```python
from build123d import *
from OCP.BRepFilletAPI import BRepFilletAPI_MakeChamfer

# Parameters (mm, degrees)
SM_BASE_FLANGE_1_DEPTH = 60
CHAMFER_2_SIZE         = 35
CHAMFER_2_SIZE2        = 15
CHAMFER_3_SIZE         = 15
CHAMFER_3_SIZE2        = 35


# Sheet-metal steps are written as plain solids
with BuildPart() as part:
    # Sketch 1 → 基体-法兰1 (new body)
    with BuildSketch(Plane(origin=(0, 0, 0), x_dir=(0, 0, -1), z_dir=(1, 0, 0))):
        with BuildLine():
            Line((-50, -25), (-27.343145751, -2.343145751))
            ThreePointArc((-27.343145751, -2.343145751), (-24.74775896, -0.60896374), (-21.686291501, 0))
            Line((-21.686291501, 0), (21.686291501, 0))
            ThreePointArc((21.686291501, 0), (24.74775896, -0.60896374), (27.343145751, -2.343145751))
            Line((27.343145751, -2.343145751), (50, -25))
            Line((50, -25), (55.656854249, -19.343145751))
            Line((55.656854249, -19.343145751), (33, 3.313708499))
            ThreePointArc((33, 3.313708499), (27.809226419, 6.78207252), (21.686291501, 8))
            Line((21.686291501, 8), (-21.686291501, 8))
            ThreePointArc((-21.686291501, 8), (-27.809226419, 6.78207252), (-33, 3.313708499))
            Line((-33, 3.313708499), (-55.656854249, -19.343145751))
            Line((-55.656854249, -19.343145751), (-50, -25))
        make_face()
    extrude(amount=SM_BASE_FLANGE_1_DEPTH)

    # 倒角2
    chamfer_2_edges = [part.edges().sort_by_distance(p)[0] for p in [
        (60, -22.171572875, 52.828427125),
        (60, -22.171572875, -52.828427125),
    ]]
    chamfer_2_side = [part.faces().sort_by_distance(p)[0] for p in [
        (60, -8.83568579, 43.50745996),
    ]]
    chamfer(chamfer_2_edges, length=CHAMFER_2_SIZE, length2=CHAMFER_2_SIZE2, reference=chamfer_2_side[0])

    # 倒角3: one chamfer whose edges measure the first distance from different faces: ONE call of the kernel's chamfer builder (chamfer() names one face for all edges)
    chamfer_3_edges_1 = [part.edges().sort_by_distance(p)[0] for p in [
        (0, -22.171572875, 52.828427125),
    ]]
    chamfer_3_side_1 = [part.faces().sort_by_distance(p)[0] for p in [
        (22.5, -22.171572875, 52.828427125),
    ]]
    chamfer_3_edges_2 = [part.edges().sort_by_distance(p)[0] for p in [
        (0, -22.171572875, -52.828427125),
    ]]
    chamfer_3_side_2 = [part.faces().sort_by_distance(p)[0] for p in [
        (22.5, -22.171572875, -52.828427125),
    ]]
    chamfer_3 = BRepFilletAPI_MakeChamfer(part.part.solid().wrapped)
    for e in chamfer_3_edges_1:
        chamfer_3.Add(CHAMFER_3_SIZE, CHAMFER_3_SIZE2, e.wrapped, chamfer_3_side_1[0].wrapped)  # the first distance lies on this face
    for e in chamfer_3_edges_2:
        chamfer_3.Add(CHAMFER_3_SIZE, CHAMFER_3_SIZE2, e.wrapped, chamfer_3_side_2[0].wrapped)  # the first distance lies on this face
    add(Compound.cast(chamfer_3.Shape()), mode=Mode.REPLACE)


solid = part.part
```
The listing builds one solid part. Answer for the finished solid, in the listing's coordinates (mm). A direction names the side the tool comes from. Give positions to 0.01 mm unless a question says otherwise; leave off trailing zeros. Order: outer loops, then holes, each group sorted by start corner. A loop starts at its lowest first (then second) coordinate and runs counter-clockwise, first axis right, second up.
Item 1: Find the intervals of material crossed by probe 1 along Y at (x, z) = (5, -1.5); probe 2 along Z at (x, y) = (22.5, -12); probe 3 along Z at (x, y) = (24, -4.5), in increasing order.
From the geometry:
probe 1: y = 0 to 8
probe 2: z = -48.31 to -37, 37 to 48.31
probe 3: z = -40.81 to -29.5, 29.5 to 40.81
Item 2: The part is cut by section B-B, the plane y = -18. Give the vertices of the cut face in (x, z).
From the geometry:
outline: (10.76, -43) - (14.19, -54.31) - (45.81, -54.31) - (49.24, -43) - close; (10.76, 43) - (49.24, 43) - (45.81, 54.31) - (14.19, 54.31) - close
Item 3: For a pull along Z with two mould halves and no side action, classify faces 3 (the face through (60, 5, 0)), 4 (the face through (30, -22, 53)), 5 (the face through (30, -11, 36)) as pulls with the +Z half, pulls with the -Z half, needs draft (parallel to the pull), parting line crosses it, or undercut.
From the geometry:
face 3: needs draft
face 4: pulls with the +Z half
face 5: undercut
Item 4: Which of the six approach directions +Z, -Z, +X, -X, +Y, -Y give full straight-line access (tool end or side, diameter ignored) to faces 1 (the face through (30, 8, 0)), 2 (the face through (30, 0, 0))?
From the geometry:
face 1: +Z, -Z, +X, -X, +Y
face 2: +X, -X, -Y
Item 5: The part is cut by section A-A, the plane x = 22. Give the vertices of the cut face in (y, z), and give its area (3 significant figures).
From the geometry:
outline: (-25, -50) - (-19.34, -55.66) - (3.31, -33) arc R16 ccw to (8, -21.69) - (8, 21.69) arc R16 ccw to (3.31, 33) - (-19.34, 55.66) - (-25, 50) - (-2.34, 27.34) arc R8 cw to (0, 21.69) - (0, -21.69) arc R8 cw to (-2.34, -27.34) - close
area: 1,010 mm2
Item 6: The part is cut by section C-C, the plane y = -6. Give the vertices of the cut face in (x, z), and give its area (3 significant figures).
From the geometry:
outline: (3.48, -31) - (6.91, -42.31) - (53.09, -42.31) - (56.52, -31) - close; (3.48, 31) - (56.52, 31) - (53.09, 42.31) - (6.91, 42.31) - close
area: 1,120 mm2
Item 7: Given pin 1 Ø3 at (x, z) = (23.5, -40) entering from -Y; pin 2 Ø1 at (x, y) = (41, -14.5) entering from +Z; pin 3 Ø3 at (x, y) = (33.5, -15.5) entering from +Z, each flat-ended and moving along its own axis, determine where each tip first touches the part or whether it passes through.
From the geometry:
pin 1: stops at y = -16.5
pin 2: stops at z = 51.31
pin 3: stops at z = 53.31
Item 8: The part is cut by section D-D, the plane z = 5. Give the vertices of the cut face in (x, y), and give its area (3 significant figures).
From the geometry:
outline: (0, 0) - (60, 0) - (60, 8) - (0, 8) - close
area: 480 mm2
